Read the model definition and answer for the solid it produces. Units are mm, in the model's axes. Face numbers are marked on the shaded views. Coordinates: 2 decimals unless noted, no trailing zeros. Write each loop counter-clockwise with the first axis right and the second up, starting at its lowest first coordinate (ties: lowest second). Pieces come first, ordered by that corner, then holes. Notation, with made-up numbers: (47, -13) -> (103, -13) arc R29 ccw to (103, 21) -> close; hole circle Ø11 at (83, 44). An arc over 180 degrees is marked (long way). One line per item, written item: value. Start each with the question number.
1. For a pull along Y with two mould halves and no side action, classify the marked faces 1, 2 and 3 as pulls with the +Y half, pulls with the -Y half, needs draft (parallel to the pull), parting line crosses it, or undercut.
2. Find section A-A, the plane x = 0. State how many separate pieces and enclosed holes the cut face has, and give its area (3 significant figures).
3. Find section C-C, the plane z = 61. Write down the section's boundary in (x, y) (1 decimal), and give its area (3 significant figures).
4. Given P1, Ø3, axis at x = -1.5, z = 79.5, coming from the -Y side (3 decimals); P2, Ø2, axis at y = 2.5, z = 13.5, coming from the +X side; P3, Ø6, axis at x = -4, z = 55, coming from the +Y side; P4, Ø3, axis at x = -2.5, y = 2, coming from the -Z side, each flat-ended and moving along its own axis, determine where each tip first touches the part or whether it passes through.
5. Consider line 1 along Z through (x, y) = (0, -8.5); line 2 along Z through (x, y) = (11, -11); line 3 along X through (y, z) = (0.5, 72.5). Determine where each line is inside the solid, lowest interval first.
```python
from build123d import *

# Parameters (mm, degrees)
SKETCH1_R               = 11.1125
SKETCH1_R_2             = 5.08
BOSS_EXTRUDE1_DEPTH     = 88.9
SKETCH4_R               = 15.875
BOSS_EXTRUDE2_DEPTH     = 19.05
CUT_EXTRUDE1_DEPTH      = 92.691009647
CUT_EXTRUDE1_DEPTH_BACK = 92.691009647
SKETCH5_R               = 3.3655
CUT_EXTRUDE2_DEPTH      = 92.691009778
CUT_EXTRUDE2_DEPTH_BACK = 92.691009778
SKETCH7_R               = 3.3655


with BuildPart() as part:
    # Sketch1 → Boss-Extrude1 (new body)
    with BuildSketch(Plane.XY):
        Circle(SKETCH1_R)
        Circle(SKETCH1_R_2, mode=Mode.SUBTRACT)
    extrude(amount=BOSS_EXTRUDE1_DEPTH)

    # Sketch4 → Boss-Extrude2 (add)
    with BuildSketch(Plane.XY.offset(88.9)):
        Circle(SKETCH4_R)
    extrude(amount=-BOSS_EXTRUDE2_DEPTH)

    # Sketch5 → Cut-Extrude1 (cut, two sides: drawn at the far end of the back side and taken through both)
    with BuildSketch(Plane(origin=(0, 0, 0), x_dir=(0, 0, -1), z_dir=(1, 0, 0)).offset(-CUT_EXTRUDE1_DEPTH_BACK)):
        with Locations((-79.375, 0)):
            Circle(SKETCH5_R)
    extrude(amount=CUT_EXTRUDE1_DEPTH + CUT_EXTRUDE1_DEPTH_BACK, mode=Mode.SUBTRACT)

    # Sketch7 → Cut-Extrude2 (cut, two sides: drawn at the far end of the back side and taken through both)
    with BuildSketch(Plane(origin=(0, 0, 0), x_dir=(1, 0, 0), z_dir=(0, 1, 0)).offset(-CUT_EXTRUDE2_DEPTH_BACK)):
        with Locations(Location((0, -9.525, 0), (0, 0, 270))):
            Circle(SKETCH7_R)
    extrude(amount=CUT_EXTRUDE2_DEPTH + CUT_EXTRUDE2_DEPTH_BACK, mode=Mode.SUBTRACT)


solid = part.part
```
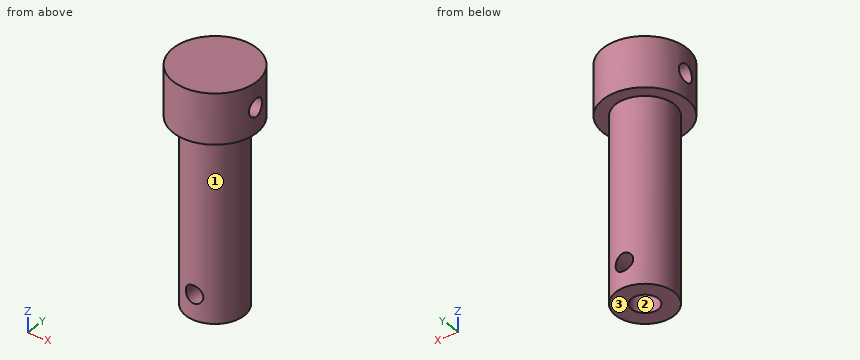
Answer block:
1. face 1: parting line crosses it
1. face 2: undercut
1. face 3: needs draft
2. separate pieces: 3
2. enclosed holes: 1
2. area: 1,330 mm2
3. outline: circle Ø22.2 at (0, 0); hole circle Ø10.2 at (0, 0)
3. area: 307 mm2
4. P1: stops at y = -15.875
4. P2: stops at x = 11.01
4. P3: stops at y = 11.07
4. P4: stops at z = 69.85
5. line 1: z = 0 to 6.16, 12.89 to 88.9
5. line 2: z = 69.85 to 88.9
5. line 3: x = -15.87 to 15.87
